Geometry check sheet. Reference: the model listing, model coordinates, mm. A direction names the side the tool comes from. Round coordinates to 2 decimals unless told otherwise and drop trailing zeros. Write each loop counter-clockwise with the first axis right and the second up, starting at its lowest first coordinate (ties: lowest second). Pieces come first, ordered by that corner, then holes. Notation, with made-up numbers: M 8,15.5 L 14,15.5 A11 ccw 14,27.5 Z; hole C -16,48 d8. An arc over 180 degrees is marked long. One line per item, written item: value. Start each with the question number.
1. Section check D-D (z = 4.5). Record the boundary of the cut face in (x, y), and give its area (3 significant figures).
2. Section check A-A (x = -45.5). Record the boundary of the cut face in (y, z).
3. Depth check by flat-ended pin: P1, Ø0.9, axis at x = 46.5, y = 0, coming from the +Z side; P2, Ø0.9, axis at y = 0.5, z = 7, coming from the +X side; P3, Ø1.5, axis at y = -0.5, z = 7, coming from the -X side. Enter the tip coordinate at first touch or a pass-through.
4. Section check B-B (z = -1.25). Record the boundary of the cut face in (x, y), and give its area (3 significant figures).
5. Section check C-C (y = -0.25). Record the boundary of the cut face in (x, z).
6. Access from +Z, -Z, +X, -X, +Y, -Y to the whole of each face (thin tool, end or side, straight path). Record for faces 5 (the flat face through (-44.5, 0, -7)), 6 (the flat face through (46, 0, 5.5)), 7 (the flat face through (46, 0, -5.5)), 8 (the flat face through (-6, 0, 5.5)), 9 (the flat face through (-44.5, 0, 7)).
7. Scan lines: probe 1 along Z at (x, y) = (18, 0.7); probe 2 along X at (y, z) = (-1.25, 6.25); probe 3 along Z at (x, y) = (39, 0). Record each from-to range of solid material in increasing order. Write a range as [from, to].
8. Release check for a two-part mould opening along X. For faces 1 (the flat face through (-3, 0, -2.5)), 2 (the flat face through (32.5, 0, -7)), 3 (the flat face through (2.5, 0, -7)), 4 (the flat face through (-52, 0, -5.5)) record: pulls with the +X half, pulls with the -X half, needs draft (parallel to the pull), parting line crosses it, or undercut.
from build123d import *

# Parameters (mm, degrees)
SKETCH1_W               = 119
SKETCH1_H               = 11
BOSS_EXTRUDE1_DEPTH     = 1.5
SKETCH2_W               = 30
SKETCH2_H               = 3
BOSS_EXTRUDE2_DEPTH     = 1.5
CUT_EXTRUDE1_DEPTH      = 61.12279102
CUT_EXTRUDE1_DEPTH_BACK = 61.12279102
SKETCH3_W               = 104
SKETCH3_H               = 5
SKETCH4_W               = 3
SKETCH4_H               = 5
BOSS_EXTRUDE3_DEPTH     = 1.5


with BuildPart() as part:
    # Sketch1 → Boss-Extrude1 (new, symmetric)
    with BuildSketch(Plane(origin=(0, 0, 0), x_dir=(1, 0, 0), z_dir=(0, 1, 0))):
        Rectangle(SKETCH1_W, SKETCH1_H)
    extrude(amount=BOSS_EXTRUDE1_DEPTH, both=True)

    # Sketch2 → Boss-Extrude2 (add, symmetric)
    with BuildSketch(Plane(origin=(0, 0, 0), x_dir=(1, 0, 0), z_dir=(0, 1, 0))):
        with Locations((-29.5, -7)):
            Rectangle(SKETCH2_W, SKETCH2_H)
        with Locations((-29.5, 7)):
            Rectangle(SKETCH2_W, SKETCH2_H)
        with Locations((17.5, -7)):
            Rectangle(SKETCH2_W, SKETCH2_H)
        with Locations((17.5, 7)):
            Rectangle(SKETCH2_W, SKETCH2_H)
    extrude(amount=BOSS_EXTRUDE2_DEPTH, both=True)

    # Sketch3 → Cut-Extrude1 (cut, two sides: drawn at the far end of the back side and taken through both)
    with BuildSketch(Plane(origin=(0, 0, 0), x_dir=(1, 0, 0), z_dir=(0, 1, 0)).offset(-CUT_EXTRUDE1_DEPTH_BACK)):
        with Locations((-2.5, 0)):
            Rectangle(SKETCH3_W, SKETCH3_H)
    extrude(amount=CUT_EXTRUDE1_DEPTH + CUT_EXTRUDE1_DEPTH_BACK, mode=Mode.SUBTRACT)

    # Sketch4 → Boss-Extrude3 (add, symmetric)
    with BuildSketch(Plane(origin=(0, 0, 0), x_dir=(1, 0, 0), z_dir=(0, 1, 0))):
        with Locations((61, 0)):
            Rectangle(SKETCH4_W, SKETCH4_H)
    extrude(amount=BOSS_EXTRUDE3_DEPTH, both=True)


solid = part.part
Result sheet:
1. outline: M -59.5,-1.5 L 59.5,-1.5 L 59.5,1.5 L -59.5,1.5 Z
1. area: 357 mm2
2. outline: M -1.5,-5.5 L 1.5,-5.5 L 1.5,-2.5 L -1.5,-2.5 Z; M -1.5,2.5 L 1.5,2.5 L 1.5,5.5 L -1.5,5.5 Z
3. P1: stops at z = 5.5
3. P2: stops at x = 32.5
3. P3: stops at x = -44.5
4. outline: M -59.5,-1.5 L -54.5,-1.5 L -54.5,1.5 L -59.5,1.5 Z; M 49.5,-1.5 L 62.5,-1.5 L 62.5,1.5 L 49.5,1.5 Z
4. area: 54.0 mm2
5. outline: M -59.5,-5.5 L -44.5,-5.5 L -44.5,-8.5 L -14.5,-8.5 L -14.5,-5.5 L 2.5,-5.5 L 2.5,-8.5 L 32.5,-8.5 L 32.5,-5.5 L 59.5,-5.5 L 59.5,-2.5 L 62.5,-2.5 L 62.5,2.5 L 59.5,2.5 L 59.5,5.5 L 32.5,5.5 L 32.5,8.5 L 2.5,8.5 L 2.5,5.5 L -14.5,5.5 L -14.5,8.5 L -44.5,8.5 L -44.5,5.5 L -59.5,5.5 Z; hole M -54.5,-2.5 L 49.5,-2.5 L 49.5,2.5 L -54.5,2.5 Z
6. face 5: -Z, -X, +Y, -Y
6. face 6: +Z, +X, +Y, -Y
6. face 7: -Z, +X, +Y, -Y
6. face 8: +Z, +Y, -Y
6. face 9: +Z, -X, +Y, -Y
7. probe 1: z = [-8.5, -2.5], [2.5, 8.5]
7. probe 2: x = [-44.5, -14.5], [2.5, 32.5]
7. probe 3: z = [-5.5, -2.5], [2.5, 5.5]
8. face 1: undercut
8. face 2: pulls with the +X half
8. face 3: undercut
8. face 4: needs draft
